For this review, take the finished solid that the model builds, in its own axes (mm). A direction names the side the tool comes from. Give positions to 0.01 mm unless a question says otherwise; leave off trailing zeros. Loops run counter-clockwise (first coordinate to the right, second up) from the corner with the lowest first, then second, coordinate; pieces in that order, holes last.
```python
from build123d import *

# Parameters (mm, degrees)
BOSS_EXTRUDE1_DEPTH = 3.175
FILLET1_R           = 80
FILLET2_R           = 8
SKETCH2_R           = 1.65
CUT_EXTRUDE1_DEPTH  = 10
CUT_EXTRUDE2_DEPTH  = 10
SKETCH4_W           = 2
SKETCH4_H           = 6
CUT_EXTRUDE3_DEPTH  = 10
CUT_EXTRUDE4_START  = -10
CUT_EXTRUDE4_DEPTH  = 10
FILLET3_R           = 15


with BuildPart() as part:
    # Sketch1 → Boss-Extrude1 (new body)
    with BuildSketch(Plane(origin=(0, 0, 0), x_dir=(1, 0, 0), z_dir=(0, 1, 0))):
        with BuildLine():
            Line((-70, 14), (-40, 14))
            Line((-40, 14), (-39.816062711, 70))
            Line((-39.816062711, 70), (-73.623466631, 79.058666579))
            ThreePointArc((-73.623466631, 79.058666579), (-83.522961568, 96.205094778), (-66.376533369, 106.104589715))
            Line((-66.376533369, 106.104589715), (0, 88.319051202))
            Line((0, 88.319051202), (66.376533369, 106.104589715))
            ThreePointArc((66.376533369, 106.104589715), (83.522961568, 96.205094778), (73.623466631, 79.058666579))
            Line((73.623466631, 79.058666579), (39.816062711, 70))
            Line((39.816062711, 70), (40, 14))
            Line((40, 14), (70, 14))
            ThreePointArc((70, 14), (84, 0), (70, -14))
            Line((70, -14), (40, -14))
            Line((40, -14), (39.816062711, -70))
            Line((39.816062711, -70), (73.623466631, -79.058666579))
            ThreePointArc((73.623466631, -79.058666579), (83.522961568, -96.205094778), (66.376533369, -106.104589715))
            Line((66.376533369, -106.104589715), (0, -88.319051202))
            Line((0, -88.319051202), (-66.376533369, -106.104589715))
            ThreePointArc((-66.376533369, -106.104589715), (-83.522961568, -96.205094778), (-73.623466631, -79.058666579))
            Line((-73.623466631, -79.058666579), (-39.816062711, -70))
            Line((-39.816062711, -70), (-40, -14))
            Line((-40, -14), (-70, -14))
            ThreePointArc((-70, -14), (-84, 0), (-70, 14))
        make_face()
    extrude(amount=BOSS_EXTRUDE1_DEPTH)

    # Fillet1
    fillet1_edges = [part.edges().sort_by_distance(p)[0] for p in [
        (0, 1.5875, -88.319051202),
        (0, 1.5875, 88.319051202),
    ]]
    fillet(fillet1_edges, radius=FILLET1_R)

    # Fillet2
    fillet2_edges = [part.edges().sort_by_distance(p)[0] for p in [
        (-40, 1.5875, -14),
        (-39.816062711, 1.5875, -70),
        (39.816062711, 1.5875, -70),
        (40, 1.5875, -14),
        (40, 1.5875, 14),
        (39.816062711, 1.5875, 70),
        (-39.816062711, 1.5875, 70),
        (-40, 1.5875, 14),
    ]]
    fillet(fillet2_edges, radius=FILLET2_R)

    # Sketch2 → Cut-Extrude1 (cut)
    with BuildSketch(Plane(origin=(0, 3.175, 0), x_dir=(1, 0, 0), z_dir=(0, 1, 0))):
        with Locations(Location((0, 87.141145635, 0), (0, 0, 270))):
            Circle(SKETCH2_R)
        with Locations(Location((-35.905030257, 42.907120147, 0), (0, 0, 270))):
            Circle(SKETCH2_R)
        with Locations(Location((35.905030257, 42.907120147, 0), (0, 0, 270))):
            Circle(SKETCH2_R)
        with Locations(Location((35.905030257, -42.907120147, 0), (0, 0, 270))):
            Circle(SKETCH2_R)
        with Locations(Location((0, -87.141145635, 0), (0, 0, 270))):
            Circle(SKETCH2_R)
        with Locations(Location((-35.905030257, -42.907120147, 0), (0, 0, 270))):
            Circle(SKETCH2_R)
    extrude(amount=-CUT_EXTRUDE1_DEPTH, mode=Mode.SUBTRACT)

    # Sketch3 → Cut-Extrude2 (cut)
    with BuildSketch(Plane(origin=(0, 3.175, 0), x_dir=(1, 0, 0), z_dir=(0, 1, 0))):
        with BuildLine():
            ThreePointArc((13.5, 26.5), (15, 25), (16.5, 26.5))
            ThreePointArc((16.5, 26.5), (15, 28), (13.5, 26.5))
        make_face()
        with BuildLine():
            ThreePointArc((-16.5, 42.5), (-15, 41), (-13.5, 42.5))
            ThreePointArc((-13.5, 42.5), (-15, 44), (-16.5, 42.5))
        make_face()
    extrude(amount=-CUT_EXTRUDE2_DEPTH, mode=Mode.SUBTRACT)

    # Sketch4 → Cut-Extrude3 (cut)
    with BuildSketch(Plane(origin=(0, 3.175, 0), x_dir=(1, 0, 0), z_dir=(0, 1, 0))):
        with Locations((-16.5, -33.141145635)):
            Rectangle(SKETCH4_W, SKETCH4_H)
        with Locations((16.5, -3.141145635)):
            Rectangle(SKETCH4_W, SKETCH4_H)
        with Locations((16.5, -33.141145635)):
            Rectangle(SKETCH4_W, SKETCH4_H)
        with Locations((-16.5, -3.141145635)):
            Rectangle(SKETCH4_W, SKETCH4_H)
    extrude(amount=-CUT_EXTRUDE3_DEPTH, mode=Mode.SUBTRACT)

    # Sketch5 → Cut-Extrude4 (cut)
    with BuildSketch(Plane(origin=(0, 3.175, 0), x_dir=(1, 0, 0), z_dir=(0, 1, 0)).offset(CUT_EXTRUDE4_START)):
        with BuildLine():
            Line((-73.623466631, 79.058666579), (-66.376533369, 106.104589715))
            ThreePointArc((-66.376533369, 106.104589715), (-83.522961568, 96.205094778), (-73.623466631, 79.058666579))
        make_face()
        with BuildLine():
            Line((73.623466631, 79.058666579), (66.376533369, 106.104589715))
            ThreePointArc((66.376533369, 106.104589715), (83.522961568, 96.205094778), (73.623466631, 79.058666579))
        make_face()
        with BuildLine():
            Line((73.623466631, -79.058666579), (66.376533369, -106.104589715))
            ThreePointArc((66.376533369, -106.104589715), (83.522961568, -96.205094778), (73.623466631, -79.058666579))
        make_face()
        with BuildLine():
            Line((-73.623466631, -79.058666579), (-66.376533369, -106.104589715))
            ThreePointArc((-66.376533369, -106.104589715), (-83.522961568, -96.205094778), (-73.623466631, -79.058666579))
        make_face()
        with BuildLine():
            Line((-70, 14), (-70, -14))
            ThreePointArc((-70, -14), (-84, 0), (-70, 14))
        make_face()
        with BuildLine():
            Line((70, 14), (70, -14))
            ThreePointArc((70, -14), (84, 0), (70, 14))
        make_face()
    extrude(amount=CUT_EXTRUDE4_DEPTH, mode=Mode.SUBTRACT)

    # Fillet3
    # the kernel refuses this fillet: 15 mm, written as the material it takes off along each edge
    with BuildSketch(Plane(origin=(66.376533369, -37.5, -106.104589715), x_dir=(0.25881904510251735, 0, 0.9659258262890692), z_dir=(0, 1, 0)), Plane(origin=(73.623466631, -37.5, -79.058666579), x_dir=(-0.9659258262890694, 0, 0.2588190451025162), z_dir=(0, 1, 0)), Plane(origin=(70, -37.5, -14), x_dir=(0, 0, 1), z_dir=(0, 1, 0)), Plane(origin=(70, -37.5, 14), x_dir=(-1, 0, 0), z_dir=(0, 1, 0)), Plane(origin=(73.623466631, -37.5, 79.058666579), x_dir=(-0.2588190451025152, 0, 0.9659258262890699), z_dir=(0, 1, 0)), Plane(origin=(66.376533369, -37.5, 106.104589715), x_dir=(-0.9659258262890692, 0, -0.2588190451025171), z_dir=(0, 1, 0)), Plane(origin=(-66.376533369, -37.5, 106.104589715), x_dir=(-0.25881904510251846, 0, -0.965925826289069), z_dir=(0, 1, 0)), Plane(origin=(-73.623466631, -37.5, 79.058666579), x_dir=(0.9659258262890696, 0, -0.25881904510251585), z_dir=(0, 1, 0)), Plane(origin=(-70, -37.5, 14), x_dir=(0, 0, -1), z_dir=(0, 1, 0)), Plane(origin=(-70, -37.5, -14), x_dir=(1, 0, 0), z_dir=(0, 1, 0)), Plane(origin=(-73.623466631, -37.5, -79.058666579), x_dir=(0.2588190451025171, 0, -0.9659258262890692), z_dir=(0, 1, 0)), Plane(origin=(-66.376533369, -37.5, -106.104589715), x_dir=(0.9659258262890688, 0, 0.2588190451025186), z_dir=(0, 1, 0))) as fillet3_piece_1:
        with BuildLine():
            CenterArc((FILLET3_R, -FILLET3_R), FILLET3_R, 90, 90)
            Line((0, -FILLET3_R), (0, 0))
            Line((0, 0), (FILLET3_R, 0))
        make_face()
    extrude(amount=78.175, mode=Mode.SUBTRACT)


solid = part.part
```
Q1. Mouldability with a two-part tool opening along X and no side actions: class faces 1 (the flat face through (-36.078, 1.565, 97.986)), 2 (the cylindrical face through (42.26, 1.61, -16.4)), 3 (the cylindrical face through (-65.13, 1.57, -10.06)) as +X half, -X half, draft (parallel to the pull), parting line (faces both ways), or undercut.
Answers:
face 1: undercut
face 2: +X half
face 3: -X half
Q2. Consider section A-A on x = -43. Give the boundary of the cut face in (y, z) (3 decimals).
Answers:
outline: (0, -99.841) - (3.175, -99.841) - (3.175, -70.239) - (0, -70.239) - close; (0, -15.734) - (3.175, -15.734) - (3.175, 15.734) - (0, 15.734) - close; (0, 70.239) - (3.175, 70.239) - (3.175, 99.841) - (0, 99.841) - close
Q3. Consider section C-C on y = 2.15. Count the separate pieces of the cut face and the enclosed holes in it, plus the area to 3 significant figures.
Answers:
separate pieces: 1
enclosed holes: 12
area: 19,600 mm2
Q4. Consider section B-B on z = 77.5. Give the boundary of the cut face in (x, y) (3 decimals).
Answers:
outline: (-64.028, 0) - (64.028, 0) - (64.028, 3.175) - (-64.028, 3.175) - close
Q5. For probe 1 along X at (y, z) = (2.55, 36); probe 2 along Z at (x, y) = (-16, 0.3); probe 3 along Z at (x, y) = (-55.5, 0.45), list the stretches that pass through material, from the lowest coordinate up.
Answers:
probe 1: x = -39.93 to -17.5, -15.5 to 15.5, 17.5 to 39.93
probe 2: z = -92.76 to -43.62, -41.38 to 0.14, 6.14 to 30.14, 36.14 to 92.76
probe 3: z = -102.73 to -74.2, -13.99 to 13.99, 74.2 to 102.73
Q6. For pin 1 Ø1 at (y, z) = (1.5, 32) entering from +X; pin 2 Ø1 at (y, z) = (2, 32.5) entering from -X; pin 3 Ø0.6 at (x, y) = (-16.5, 2) entering from +Z, all flat-tipped, find the tip position at first contact; note any pin that passes through.
Answers:
pin 1: stops at x = 39.94
pin 2: stops at x = -39.94
pin 3: stops at z = 92.93
Q7. Machinability: for faces 4 (the cylindrical face through (-42.26, 1.61, -16.4)), 5 (the flat face through (-36.5, 1.6, -98.1)), 6 (the cylindrical face through (41.44, 1.61, 68.67)), which of the approach directions +Z, -Z, +X, -X, +Y, -Y give a long, thin tool a straight path to every point of the face, cutting with its end or side? Answer none if there is none.
Answers:
face 4: -X, +Y, -Y
face 5: -Z, +Y, -Y
face 6: +X, +Y, -Y
